Build history of the part. All positions in model axes, mm. A direction names the side the tool comes from. Round coordinates to 2 decimals unless told otherwise and drop trailing zeros. Write each loop counter-clockwise with the first axis right and the second up, starting at its lowest first coordinate (ties: lowest second). Pieces come first, ordered by that corner, then holes. Notation, with made-up numbers: M 9.5,23 L 29.5,23 A27 cw 29.5,41 Z; hole C -21.5,32 d6. An arc over 180 degrees is marked long. Write item = value, one per line. Start each with the question number.
Q1. Drop flat-ended pins along their axis: P1, Ø2, axis at x = 12.5, y = 20, coming from the -Z side; P2, Ø10, axis at x = -26.5, z = -16.5, coming from the +Y side; P3, Ø19, axis at x = -2, y = -8.5, coming from the +Z side. Give the stop position or say it passes through.
Q2. Band-saw the part on B-B on x = 3. Write the cut outline in (y, z).
Q3. Band-saw the part on A-A on z = -13.5. Write the cut outline in (x, y).
Q4. Pull direction X, two halves, no side cores. Call faces 1 (the flat face through (-15, -5, 0)), 2 (the cylindrical face through (-14.03, 18.58, 11.99)), 3 (the flat face through (-15, -5, 8.879)): released by +X, released by -X, zero draft, split by the parting line, or undercut.
Q5. Band-saw the part on C-C on y = -8.5. Write the cut outline in (x, z), plus the area to 3 significant figures.
Q6. Tool access for faces 4 (the cylindrical face through (-44.173, -30.562, -13.63)), 5 (the flat face through (-47, 17, -25.4)), 6 (the flat face through (-30, -31, -25.4)): list every direction of +Z, -Z, +X, -X, +Y, -Y with a clear straight run to the whole face (end or side of a thin tool).
Q7. Band-saw the part on D-D on z = 10. Write the cut outline in (x, y), plus the area to 3 significant figures.
Q8. Probe L1, parallel to Z at x = -46, y = 4.5; L2, parallel to X at y = 11, z = -1.5; L3, parallel to Y at x = -45, z = -16. List the from-to ranges inside material, lowest first.
```python
from build123d import *

# Parameters (mm, degrees)
F0_W      = 76.2
F0_H      = 63.5
F1_DEPTH  = 8.87915
F2_R      = 3.2312727432
F3_DEPTH  = 27.64789
F2_R_2    = 3.4736024705
F2_R_3    = 3.4228960701
F2_R_4    = 3.2312730123
F4_DEPTH  = 25.4
F5_R      = 3.9275858197
F5_R_2    = 3.4275613836
F6_DEPTH  = 6.31556
F9_R      = 4.0783648595
F9_R_2    = 3.9191806832
F9_R_3    = 3.5394300608
F9_R_4    = 3.4524766022
F10_DEPTH = 25.4


# Not quite as in the source:
# - the program builds the solid bodies; features that only make, move or delete a surface that nothing else refers to are left out


with BuildPart() as f1:
    # F0 (on Top) → F1 (new body)
    with BuildSketch(Plane.XY):
        with Locations((-14.3929980695, -5.2504202625)):
            Rectangle(F0_W, F0_H)
    extrude(amount=F1_DEPTH)

    # F2 (on face) → F3 (join)
    with BuildSketch(Plane(origin=(0, 0, 0), x_dir=(1, 0, 0), z_dir=(0, 0, -1))):
        with Locations((-47.1578612924, 31.7992158234)):
            Circle(F2_R)
    extrude(amount=F3_DEPTH)

    # F2 (on face) → F4 (join)
    with BuildSketch(Plane(origin=(0, 0, 0), x_dir=(1, 0, 0), z_dir=(0, 0, -1))):
        with Locations((-47.1578612924, 31.7992158234)):
            Circle(F2_R)
        with Locations((-47.1578612924, -17.4867473543)):
            Circle(F2_R_2)
        with Locations((14.2814768478, -18.8030768186)):
            Circle(F2_R_3)
        with Locations((15.0982076302, 31.1281010509)):
            Circle(F2_R_4)
    extrude(amount=F4_DEPTH)

    # F5 (on face) → F6 (join)
    with BuildSketch(Plane.XY.offset(8.87915)):
        with Locations((-15.6099880114, -31.4252711833)):
            Circle(F5_R)
        with Locations((-15.6099880114, 21.6196272522)):
            Circle(F5_R_2)
    extrude(amount=F6_DEPTH)

    # F9 (on face) → F10 (join)
    with BuildSketch(Plane(origin=(0, 0, 0), x_dir=(1, 0, 0), z_dir=(0, 0, -1))):
        with Locations((-5.5510420352, -13.5985026136)):
            Circle(F9_R)
        with Locations((-28.7904683501, -13.2877733558)):
            Circle(F9_R_2)
        with Locations((-29.9201626331, 31.2515720725)):
            Circle(F9_R_3)
        with Locations((-6.5234871581, 32.5696654618)):
            Circle(F9_R_4)
    extrude(amount=F10_DEPTH)


solid = f1.part
```
Conclusion:
q1.P1 = -25.4
q1.P2 = 17.21
q1.P3 = 8.88
q2.outline = M -37,0 L 26.5,0 L 26.5,8.88 L -37,8.88 Z
q3.outline = C -47.16,17.49 d6.95; C -47.16,-31.8 d6.46; C -29.92,-31.25 d7.08; C -28.79,13.29 d7.84; C -6.52,-32.57 d6.9; C -5.55,13.6 d8.16; C 14.28,18.8 d6.85; C 15.1,-31.13 d6.46
q4.face_1 = undercut
q4.face_2 = split by the parting line
q4.face_3 = zero draft
q5.outline = M -52.49,0 L 23.71,0 L 23.71,8.88 L -52.49,8.88 Z
q5.area = 677 mm^2
q6.face_4 = -Z
q6.face_5 = -Z, +X, -X, +Y
q6.face_6 = -Z, +X, +Y, -Y
q7.outline = C -15.61,-31.43 d7.86; C -15.61,21.62 d6.86
q7.area = 85.4 mm^2
q8.L1 = 0 to 8.88
q8.L2 = -31.97 to -25.61, -8.69 to -2.41
q8.L3 = -34.2 to -29.39, 14.76 to 20.21
